Geometry check sheet. Reference: the model listing, model coordinates, mm. Face numbers are marked on the shaded views. A direction names the side the tool comes from. Coordinates: 2 decimals unless noted, no trailing zeros. Loops run counter-clockwise (first coordinate to the right, second up) from the corner with the lowest first, then second, coordinate; pieces in that order, holes last. Notation, with made-up numbers: M 83.5,70 L 91.5,70 A15 ccw 91.5,78 Z; hole C -21.5,21 d6. An arc over 180 degrees is marked long. Use CSV: the item, a comma, the result in double quotes.
```python
from build123d import *

# Parameters (mm, degrees)
F2_R          = 8
F3_DEPTH      = 5.116
F3_DEPTH_BACK = 5.116
F4_R          = 8
F4_R_2        = 7
F5_DEPTH      = 0.5


with BuildPart() as f1:
    # F0 (on Front) → F1 (revolve)
    with BuildSketch(Plane.XZ):
        Polygon((9.77, 5.115), (0, 5.115), (0, -5.115), (9.77, -5.115), (11.945, -2.94), (11.945, 2.94), align=None)
    revolve(axis=Axis((0, 0, 0), (0, 0, -1)))

    # F2 (on Top) → F3 (cut, two sides)
    with BuildSketch(Plane.XY) as f3_sk:
        Circle(F2_R)
    extrude(amount=-F3_DEPTH, mode=Mode.SUBTRACT)
    extrude(f3_sk.sketch, amount=F3_DEPTH_BACK, mode=Mode.SUBTRACT)

    # F4 (on Top) → F5 (join, symmetric)
    with BuildSketch(Plane.XY):
        Circle(F4_R)
        Circle(F4_R_2, mode=Mode.SUBTRACT)
    extrude(amount=F5_DEPTH, both=True)


solid = f1.part
```
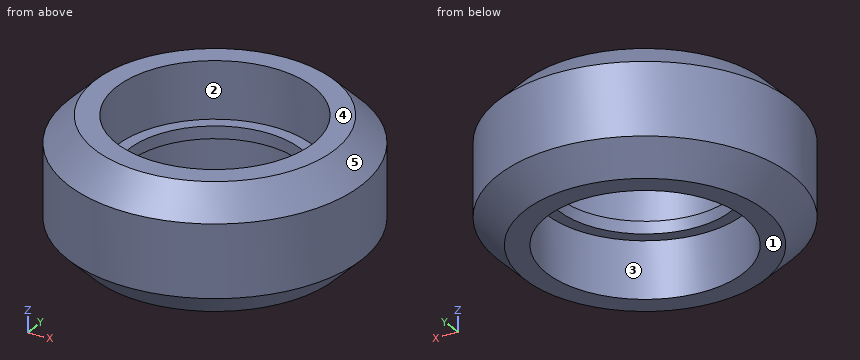
1. Thickness scan on line 1 (X direction, y = 0, z = 2.25) (3 decimals); line 2 (X direction, y = 2.5, z = 2); line 3 (Z direction, x = -2.5, y = 6.75). Record the ranges inside material, lowest first. Write a range as [from, to].
The answers:
line 1,"[-11.945, -8], [8, 11.945]"
line 2,"[-11.68, -7.6], [7.6, 11.68]"
line 3,"[-0.5, 0.5]"
2. Section check D-D, the plane z = -3.75. Record the cut outline in (x, y) (3 decimals).
The answers:
outline,"C 0,0 d22.27; hole C 0,0 d16"
3. Section check A-A, the plane y = 0. Record the cut outline in (x, z) (3 decimals).
The answers:
outline,"M -11.945,-2.94 L -9.77,-5.115 L -8,-5.115 L -8,-0.5 L -7,-0.5 L -7,0.5 L -8,0.5 L -8,5.115 L -9.77,5.115 L -11.945,2.94 Z; M 7,-0.5 L 8,-0.5 L 8,-5.115 L 9.77,-5.115 L 11.945,-2.94 L 11.945,2.94 L 9.77,5.115 L 8,5.115 L 8,0.5 L 7,0.5 Z"
4. Section check C-C, the plane z = 1.75. Record the cut outline in (x, y) (3 decimals), plus the area to 3 significant figures.
The answers:
outline,"C 0,0 d23.89; hole C 0,0 d16"
area,"247 mm^2"
5. Set-up check for the marked faces 1 and 2: record each of +Z, -Z, +X, -X, +Y, -Y from which the full face is reachable in a straight line by a thin tool's end or side.
The answers:
face 1,"-Z, +X, -X, +Y, -Y"
face 2,"+Z"
6. Gauge pin test, flat ends, axial feed: P1, Ø5, axis at x = -8, y = -6.5, coming from the +Z side (3 decimals); P2, Ø1.5, axis at x = -0.5, z = 4, coming from the -Y side; P3, Ø5, axis at y = 4.5, z = -2.5, coming from the +X side; P4, Ø6, axis at x = -5.5, z = 3.5, coming from the +Y side. Record the tip position at first contact, or that the pin passes through.
The answers:
P1,"z = 5.115"
P2,"y = -11.62"
P3,"x = 11.78"
P4,"y = 11.67"
7. Release check for a two-part mould opening along Y. For the marked faces 3, 4 and 5 record: +Y half, -Y half, draft (parallel to the pull), parting line (faces both ways), or undercut.
The answers:
face 3,"undercut"
face 4,"draft"
face 5,"parting line"
